Geometry check sheet. Reference: the model listing, model coordinates, mm. A direction names the side the tool comes from. Give positions to 0.01 mm unless a question says otherwise; leave off trailing zeros. Write each loop counter-clockwise with the first axis right and the second up, starting at its lowest first coordinate (ties: lowest second). Pieces come first, ordered by that corner, then holes. Notation, with made-up numbers: (34.25, 59) - (88.25, 59) arc R10 cw to (88.25, 65) - close; hole circle Ø1 at (87.5, 73.5). An arc over 180 degrees is marked (long way). Write item = value, one per line. Start each with the question number.
(1) Section check A-A, the plane x = 10.5. Enter the section's corners in (y, z).
(2) Thickness scan on L1, parallel to X at y = 3, z = -24; L2, parallel to Y at x = -21, z = -23.6; L3, parallel to Z at x = 28.5, y = 14.5. Record the ranges inside material, lowest first.
(3) Depth check by flat-ended pin: pin 1 Ø17.5 at (x, y) = (8.5, 33) entering from -Z; pin 2 Ø5 at (x, z) = (25.5, 17.5) entering from -Y. Enter the tip coordinate at first touch or a pass-through.
(4) Section check C-C, the plane x = -18. Enter the section's corners in (y, z).
(5) Section check D-D, the plane z = 15. Enter the section's corners in (x, y), plus the area to 3 significant figures.
(6) Draft check along X on faces 4 (the flat face through (-3, 58, 24)), 5 (the cylindrical face through (-19.43, 2.35, -23.97)). Enter one of: pulls with the +X half, pulls with the -X half, needs draft (parallel to the pull), parting line crosses it, or undercut.
(7) Access from +Z, -Z, +X, -X, +Y, -Y to the whole of each face (thin tool, end or side, straight path). Record for faces 1 (the flat face through (0, 54, -24)), 2 (the flat face through (30, 51.5, -16)), 3 (the flat face through (19, 29, -23)).
(8) Section check B-B, the plane y = 34.5. Enter the section's corners in (x, z).
```python
from build123d import *

# Parameters (mm, degrees)
SKETCH_1_W                   = 64
SKETCH_1_H                   = 50
EXTRUDE_2_DEPTH              = 58
SKETCH_2_W                   = 58
SKETCH_2_H                   = 46
CUT_EXTRUDE_1_DEPTH          = 71.802542327
SKETCH_5_W                   = 2
SKETCH_5_H                   = 45
CUT_EXTRUDE_2_DEPTH          = 50
SKETCH_6_W                   = 2
SKETCH_6_H                   = 45
CUT_EXTRUDE_3_DEPTH          = 50
HOLE_WIZARD_M3_1_D           = 3.4
HOLE_WIZARD_M3_1_DEPTH       = 5
HOLE_WIZARD_M3_1_CSINK_D     = 3.45
HOLE_WIZARD_M3_1_CSINK_ANGLE = 90
HOLE_WIZARD_M3_1_TIP         = 1.021463052
SKETCH_9_W                   = 30
SKETCH_9_H                   = 50
CUT_EXTRUDE_4_DEPTH          = 30


with BuildPart() as part:
    # 草图1 → 凸台-拉伸2 (new body)
    with BuildSketch(Plane(origin=(0, 0, 0), x_dir=(1, 0, 0), z_dir=(0, 1, 0))):
        Rectangle(SKETCH_1_W, SKETCH_1_H)
    extrude(amount=EXTRUDE_2_DEPTH)

    # 草图2 → 切除-拉伸1 (cut, through all)
    with BuildSketch(Plane.XZ):
        Rectangle(SKETCH_2_W, SKETCH_2_H)
    extrude(amount=-CUT_EXTRUDE_1_DEPTH, mode=Mode.SUBTRACT)

    # 草图5 → 切除-拉伸2 (cut)
    with BuildSketch(Plane.ZY.offset(-29)):
        with Locations((-16, 29)):
            Rectangle(SKETCH_5_W, SKETCH_5_H)
    extrude(amount=-CUT_EXTRUDE_2_DEPTH, mode=Mode.SUBTRACT)

    # 草图6 → 切除-拉伸3 (cut)
    with BuildSketch(Plane(origin=(-29, 0, 0), x_dir=(0, 0, -1), z_dir=(1, 0, 0))):
        with Locations((16, 29)):
            Rectangle(SKETCH_6_W, SKETCH_6_H)
    extrude(amount=-CUT_EXTRUDE_3_DEPTH, mode=Mode.SUBTRACT)

    # M3 间隙孔1
    with Locations(Plane(origin=(0, 0, -25), x_dir=(-1, 0, 0), z_dir=(0, 0, -1))):
        with Locations((-21, 55), (-21, 3), (21, 3), (21, 55)):
            CounterSinkHole(HOLE_WIZARD_M3_1_D / 2, HOLE_WIZARD_M3_1_CSINK_D / 2, depth=HOLE_WIZARD_M3_1_DEPTH, counter_sink_angle=HOLE_WIZARD_M3_1_CSINK_ANGLE)
            with Locations((0, 0, -(HOLE_WIZARD_M3_1_DEPTH + HOLE_WIZARD_M3_1_TIP / 2))):  # 118° drill point
                Cone(0, HOLE_WIZARD_M3_1_D / 2, HOLE_WIZARD_M3_1_TIP, mode=Mode.SUBTRACT)

    # 草图9 → 切除-拉伸4 (cut)
    with BuildSketch(Plane(origin=(0, 0, -25), x_dir=(-1, 0, 0), z_dir=(0, 0, -1))):
        with Locations((0, 29)):
            Rectangle(SKETCH_9_W, SKETCH_9_H)
    extrude(amount=-CUT_EXTRUDE_4_DEPTH, mode=Mode.SUBTRACT)


solid = part.part
```
Model answer:
q1.outline = (0, -25) - (4, -25) - (4, -23) - (0, -23) - close; (0, 23) - (58, 23) - (58, 25) - (0, 25) - close; (54, -25) - (58, -25) - (58, -23) - (54, -23) - close
q2.L1 = -32 to -22.7, -19.3 to 19.3, 22.7 to 32
q2.L2 = 0 to 1.3, 4.7 to 53.3, 56.7 to 58
q2.L3 = -25 to -23, 23 to 25
q3.pin_1 = -25
q3.pin_2 = through
q4.outline = (0, -25) - (58, -25) - (58, -23) - (0, -23) - close; (0, 23) - (58, 23) - (58, 25) - (0, 25) - close
q5.outline = (-32, 0) - (-29, 0) - (-29, 58) - (-32, 58) - close; (29, 0) - (32, 0) - (32, 58) - (29, 58) - close
q5.area = 348 mm²
q6.face_4 = needs draft
q6.face_5 = undercut
q7.face_1 = -Z
q7.face_2 = +X, -X
q7.face_3 = +Y, -Y
q8.outline = (-32, -25) - (-15, -25) - (-15, -23) - (-29, -23) - (-29, -17) - (-32, -17) - close; (-32, -15) - (-29, -15) - (-29, 23) - (29, 23) - (29, -15) - (32, -15) - (32, 25) - (-32, 25) - close; (15, -25) - (32, -25) - (32, -17) - (29, -17) - (29, -23) - (15, -23) - close
